Print and shaded views of the part. All mm, measured from the part's lowest x, y and z. A direction names the side the tool comes from. Give positions to 0.01 mm unless a question says otherwise; leave off trailing zeros. Write each loop counter-clockwise with the first axis right and the second up, starting at its lowest first coordinate (ties: lowest second). Pieces come first, ordered by that corner, then holes. Notation, with made-up numbers: (50, -12.75) - (78, -12.75) arc R12 ccw to (78, -3.75) - close; hole circle Ø5 at (64, 14.5). An arc over 180 degrees is marked (long way). Use one line per item in the form item = value. Start each with the question number.
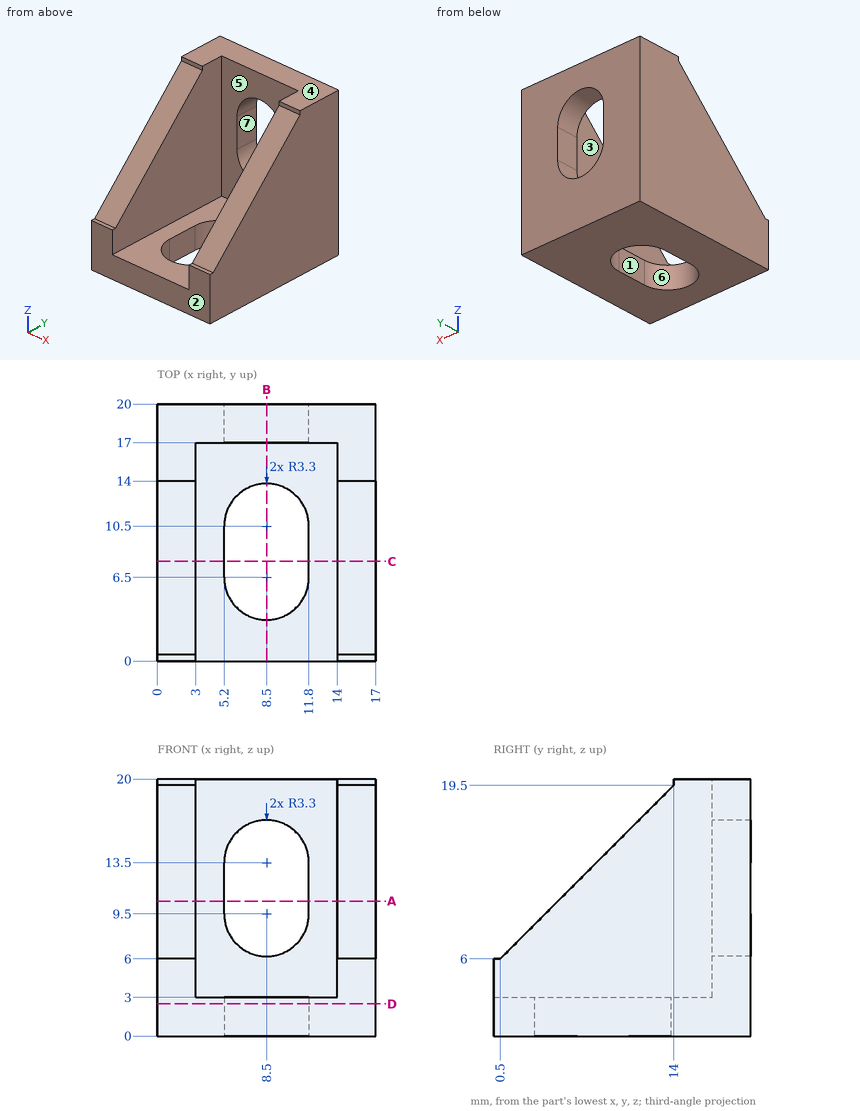
(1) Two-plate mould, pull along Y, no slides. Class the marked faces 1, 2 and 3: +Y half, -Y half, draft (parallel to the pull), parting line (faces both ways), or undercut.
(2) Wall check: line 1 (X direction, y = 10, z = 9.5); line 2 (Y direction, x = 3.25, z = 5.75); line 3 (Z direction, x = 3.25, y = 1.5). Give the ranges that are in metal, low to high. Write a range as from..to.
(3) Pin check, flat tips, straight feed: pin 1 Ø0.6 at (x, z) = (15.5, 20) entering from -Y; pin 2 Ø3.5 at (x, y) = (10, 6) entering from +Z; pin 3 Ø8 at (x, y) = (10.5, 4) entering from +Z. Stop position of each tip, or through.
(4) Cut at C-C, the plane y = 7.75. Give the cut face in (x, z).
(5) Cut at A-A, the plane z = 10.5. Give the cut face in (x, y), then the cut area to 3 significant figures.
(6) Cut at B-B, the plane x = 8.5. Give the cut face in (y, z), then the cut area to 3 significant figures.
(7) Cut at D-D, the plane z = 2.5. Give the cut face in (x, y), then the cut area to 3 significant figures.
(8) Which spindle directions (+Z, -Z, +X, -X, +Y, -Y) get a long thin tool onto all of the face, cutting with end or side? Do the marked faces 4, 5, 6 and 7. Say none if no direction does.
Solution:
q1.face_1 = undercut
q1.face_2 = -Y half
q1.face_3 = draft
q2.line_1 = 0..3, 14..17
q2.line_2 = 17..20
q2.line_3 = 0..3
q3.pin_1 = 14
q3.pin_2 = 3
q3.pin_3 = 11.44
q4.outline = (0, 0) - (5.2, 0) - (5.2, 3) - (3, 3) - (3, 13.25) - (0, 13.25) - close; (11.8, 0) - (17, 0) - (17, 13.25) - (14, 13.25) - (14, 3) - (11.8, 3) - close
q5.outline = (0, 5) - (3, 5) - (3, 17) - (5.2, 17) - (5.2, 20) - (0, 20) - close; (11.8, 17) - (14, 17) - (14, 5) - (17, 5) - (17, 20) - (11.8, 20) - close
q5.area = 103 mm2
q6.outline = (0, 0) - (3.2, 0) - (3.2, 3) - (0, 3) - close; (13.8, 0) - (20, 0) - (20, 6.2) - (17, 6.2) - (17, 3) - (13.8, 3) - close; (17, 16.8) - (20, 16.8) - (20, 20) - (17, 20) - close
q6.area = 47.4 mm2
q7.outline = (0, 0) - (17, 0) - (17, 20) - (0, 20) - close; hole (5.2, 6.5) arc R3.3 ccw to (11.8, 6.5) - (11.8, 10.5) arc R3.3 ccw to (5.2, 10.5) - close
q7.area = 279 mm2
q8.face_4 = +Z, +X, -X, +Y, -Y
q8.face_5 = +Z, -Y
q8.face_6 = +Z, -Z
q8.face_7 = +Y, -Y
